Answer from the drawing. Dimensions are ordinates in mm from the lowest x, y and z of the part. Coordinates: 2 decimals unless noted, no trailing zeros. Write each loop counter-clockwise with the first axis right and the second up, starting at its lowest first coordinate (ties: lowest second). Pieces come first, ordered by that corner, then holes. Notation, with made-up numbers: (25, 38) - (36, 38) arc R19 cw to (36, 46) - close; hole circle Ø6 at (39, 56). An arc over 180 degrees is marked (long way). Return JSON: item names as keys, results as strings.
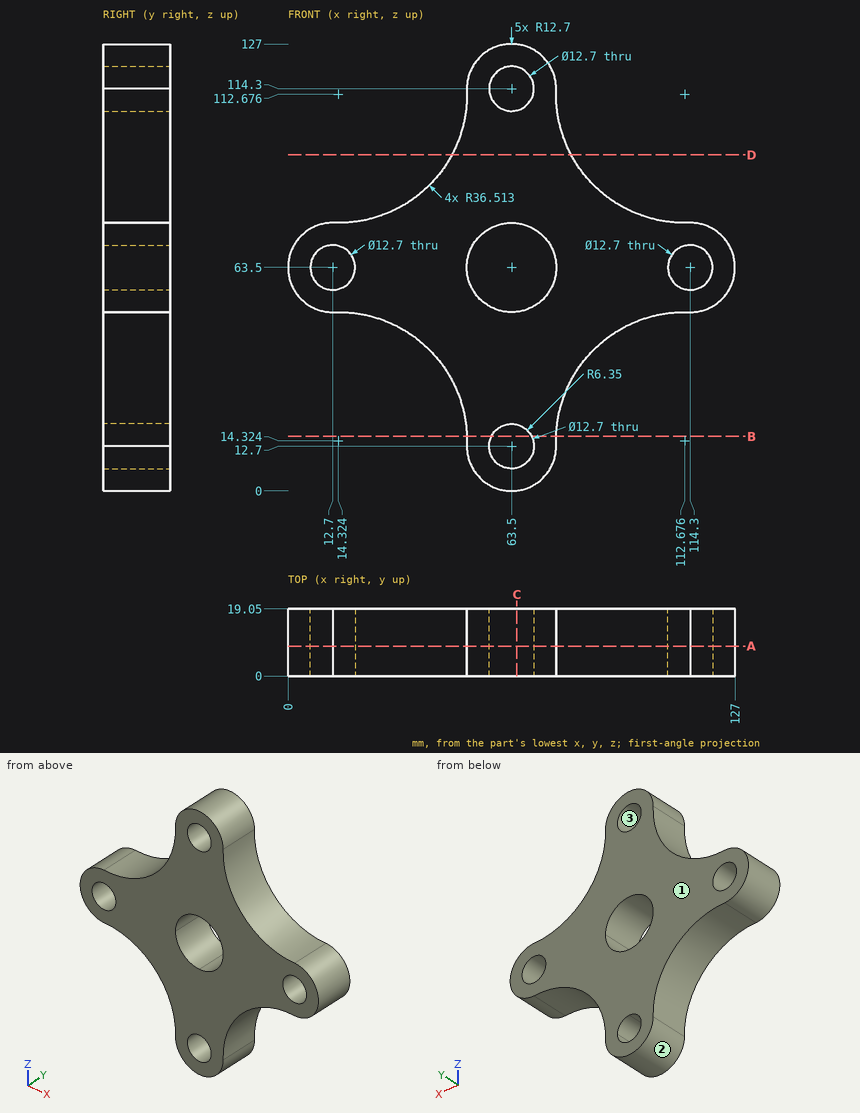
(1) Flat-ended cylindrical pins translate along their axes: P1, Ø2, axis at y = 15, z = 21.5, coming from the -X side; P2, Ø1.5, axis at y = 9.5, z = 17.5, coming from the -X side (1 decimal); P3, Ø2, axis at y = 12, z = 81.5, coming from the -X side (1 decimal). Find the tip coordinate at first contact, or state that the pin passes through.
Answer:
{"P1": "x = 49.91", "P2": "x = 50.6", "P3": "x = 31.6"}
(2) Straight lines are drawn through the part: line 1 (Z direction, x = 63.5, y = 5); line 2 (X direction, y = 4.25, z = 67.5) (1 decimal); line 3 (Z direction, x = 114.3, y = 8.25). For each, find the intervals that lie inside material, in ascending order. Write a range as from..to.
Answer:
{"line 1": "0..6.35, 19.05..50.8, 76.2..107.95, 120.65..127", "line 2": "0.6..7.8, 17.6..51.4, 75.6..109.4, 119.2..126.4", "line 3": "50.8..57.15, 69.85..76.2"}
(3) A cutting plane is placed at D-D (z = 95.5). Determine the outline of the cut face in (x, y).
Answer:
{"outline": "(46.54, 0) - (80.46, 0) - (80.46, 19.05) - (46.54, 19.05) - close"}
(4) Determine the mould class of the marked faces 1, 2 and 3 for opening direction X: +X half, -X half, draft (parallel to the pull), parting line (faces both ways), or undercut.
Answer:
{"face 1": "draft", "face 2": "parting line", "face 3": "undercut"}
(5) A cutting plane is placed at C-C (x = 65). Determine the outline of the cut face in (y, z).
Answer:
{"outline": "(0, 0.09) - (19.05, 0.09) - (19.05, 6.53) - (0, 6.53) - close; (0, 18.87) - (19.05, 18.87) - (19.05, 50.89) - (0, 50.89) - close; (0, 76.11) - (19.05, 76.11) - (19.05, 108.13) - (0, 108.13) - close; (0, 120.47) - (19.05, 120.47) - (19.05, 126.91) - (0, 126.91) - close"}
(6) A cutting plane is placed at B-B (z = 15.5). Determine the outline of the cut face in (x, y).
Answer:
{"outline": "(50.82, 0) - (57.8, 0) - (57.8, 19.05) - (50.82, 19.05) - close; (69.2, 0) - (76.18, 0) - (76.18, 19.05) - (69.2, 19.05) - close"}
(7) A cutting plane is placed at A-A (y = 8.5). State how many separate pieces and enclosed holes the cut face has, and give its area (3 significant figures).
Answer:
{"separate pieces": "1", "enclosed holes": "5", "area": "5,650 mm²"}
